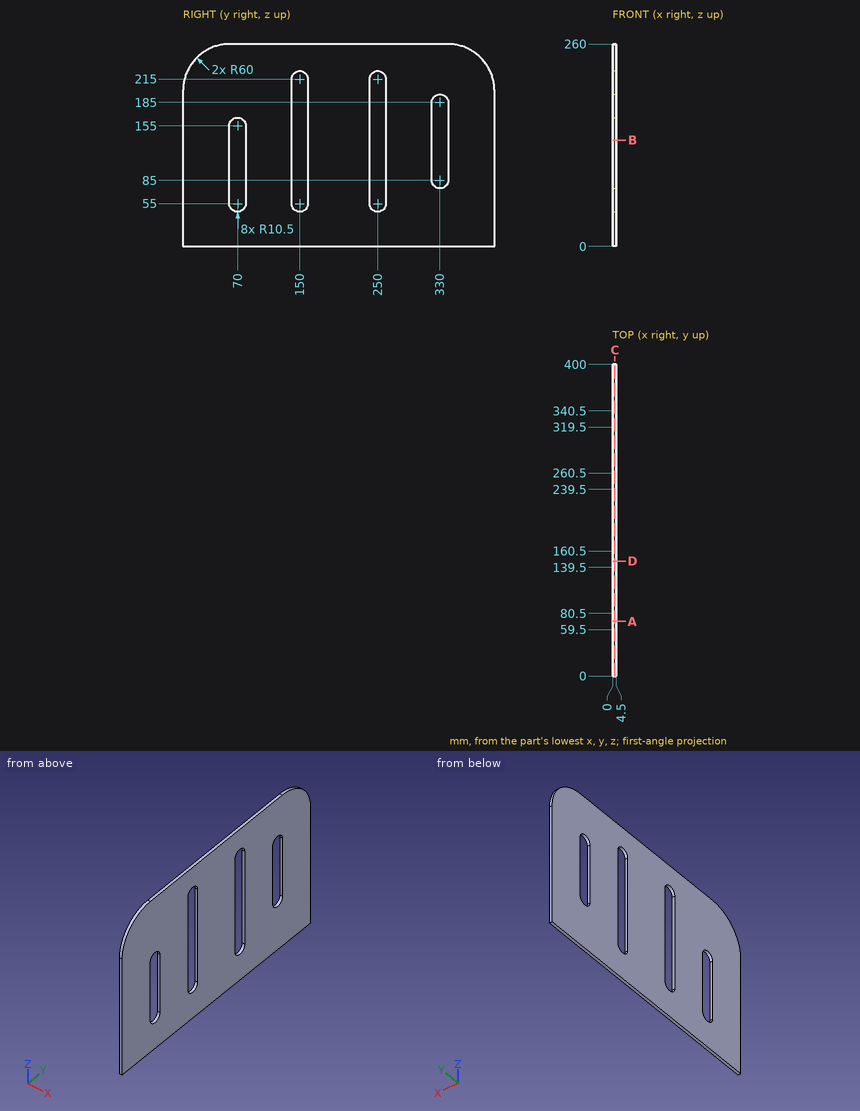
Job drawing, mm, ordinate dimensions from the low corner. One solid piece. Coordinates: 2 decimals unless noted, no trailing zeros. Write each loop counter-clockwise with the first axis right and the second up, starting at its lowest first coordinate (ties: lowest second). Pieces come first, ordered by that corner, then holes. Notation, with made-up numbers: (-32, 81) -> (10, 81) arc R14 ccw to (10, 108) -> close; hole circle Ø5 at (2, -15.5). An arc over 180 degrees is marked (long way). Use CSV: the item, a comma, the result in double quotes. Start each with the question number.
Item 1: Wall check: probe 1 along Y at (x, z) = (0.8, 115.5); probe 2 along Y at (x, z) = (2.2, 59); probe 3 along Y at (x, z) = (3.1, 179). Give the ranges that are in metal, low to high.
Item 2: Drop a flat-ended pin along its axis: P1, Ø1, axis at y = 175.5, z = 87.5, coming from the -X side. Give the stop position or say it passes through.
Item 3: Band-saw the part on C-C, the plane x = 3.15. Write the cut outline in (y, z).
Item 4: Band-saw the part on A-A, the plane y = 70. Write the cut outline in (x, z).
Item 5: Band-saw the part on B-B, the plane z = 136.5. Write the cut outline in (x, y).
Item 6: Band-saw the part on D-D, the plane y = 147.5. Write the cut outline in (x, z).
Response values:
1,probe 1,"y = 0 to 59.5, 80.5 to 139.5, 160.5 to 239.5, 260.5 to 319.5, 340.5 to 400"
1,probe 2,"y = 0 to 59.5, 80.5 to 139.5, 160.5 to 239.5, 260.5 to 400"
1,probe 3,"y = 0 to 139.5, 160.5 to 239.5, 260.5 to 319.5, 340.5 to 400"
2,P1,"stops at x = 0"
3,outline,"(0, 0) -> (400, 0) -> (400, 200) arc R60 ccw to (340, 260) -> (60, 260) arc R60 ccw to (0, 200) -> close; hole (59.5, 55) arc R10.5 ccw to (80.5, 55) -> (80.5, 155) arc R10.5 ccw to (59.5, 155) -> close; hole (139.5, 55) arc R10.5 ccw to (160.5, 55) -> (160.5, 215) arc R10.5 ccw to (139.5, 215) -> close; hole (239.5, 55) arc R10.5 ccw to (260.5, 55) -> (260.5, 215) arc R10.5 ccw to (239.5, 215) -> close; hole (319.5, 85) arc R10.5 ccw to (340.5, 85) -> (340.5, 185) arc R10.5 ccw to (319.5, 185) -> close"
4,outline,"(0, 0) -> (4.5, 0) -> (4.5, 44.5) -> (0, 44.5) -> close; (0, 165.5) -> (4.5, 165.5) -> (4.5, 260) -> (0, 260) -> close"
5,outline,"(0, 0) -> (4.5, 0) -> (4.5, 59.5) -> (0, 59.5) -> close; (0, 80.5) -> (4.5, 80.5) -> (4.5, 139.5) -> (0, 139.5) -> close; (0, 160.5) -> (4.5, 160.5) -> (4.5, 239.5) -> (0, 239.5) -> close; (0, 260.5) -> (4.5, 260.5) -> (4.5, 319.5) -> (0, 319.5) -> close; (0, 340.5) -> (4.5, 340.5) -> (4.5, 400) -> (0, 400) -> close"
6,outline,"(0, 0) -> (4.5, 0) -> (4.5, 44.8) -> (0, 44.8) -> close; (0, 225.2) -> (4.5, 225.2) -> (4.5, 260) -> (0, 260) -> close"
